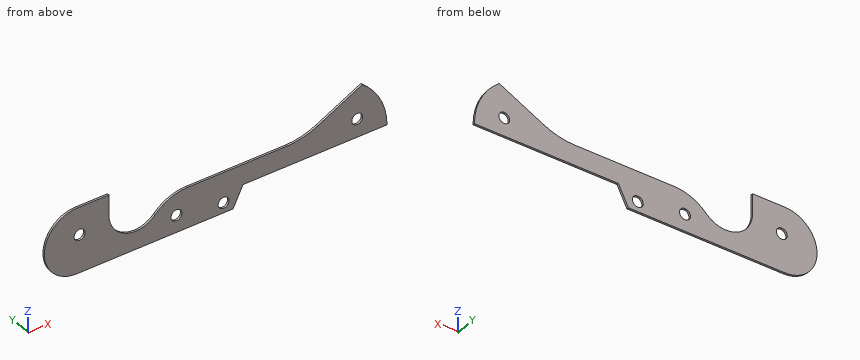
```python
from build123d import *

# Parameters (mm, degrees)
BOSS_EXTRUDE1_DEPTH = 0.508
SKETCH2_R           = 1.397
CUT_EXTRUDE1_DEPTH  = 1.508


with BuildPart() as part:
    # Sketch1 → Boss-Extrude1 (new body)
    with BuildSketch(Plane(origin=(0, 0, 0), x_dir=(1, 0, 0), z_dir=(0, 1, 0))):
        with BuildLine():
            Line((0, 8.255), (40.005, 8.255))
            Line((40.005, 8.255), (42.545, 3.175))
            Line((42.545, 3.175), (79.375, 3.175))
            ThreePointArc((79.375, 3.175), (77.699031657, -3.924515829), (73.025, -9.525))
            Line((73.025, -9.525), (61.684438597, -3.808211822))
            ThreePointArc((61.684438597, -3.808211822), (57.789960212, -2.38631827), (53.672063189, -1.905))
            Line((53.672063189, -1.905), (28.272063189, -1.905))
            ThreePointArc((28.272063189, -1.905), (23.804442177, -0.995706369), (20.047648696, 1.5875))
            ThreePointArc((20.047648696, 1.5875), (12.544893378, 3.184008757), (8.255, -3.175))
            Line((8.255, -3.175), (8.255, -8.255))
            Line((8.255, -8.255), (0, -8.255))
            ThreePointArc((0, -8.255), (-8.255, 0), (0, 8.255))
        make_face()
    extrude(amount=BOSS_EXTRUDE1_DEPTH)

    # Sketch2 → Cut-Extrude1 (cut, through all)
    with BuildSketch(Plane(origin=(0, 0.508, 0), x_dir=(1, 0, 0), z_dir=(0, 1, 0))):
        with Locations((0.762, -1.27)):
            Circle(SKETCH2_R)
        with Locations((25.527, 3.937)):
            Circle(SKETCH2_R)
        with Locations((37.592, 5.715)):
            Circle(SKETCH2_R)
        with Locations((71.755, -1.397)):
            Circle(SKETCH2_R)
    extrude(amount=-CUT_EXTRUDE1_DEPTH, mode=Mode.SUBTRACT)


solid = part.part
```
Source: CAD feature listing. Evaluate the final solid. Frame: model axes, mm. Coordinates: 2 decimals unless noted, no trailing zeros. Write each loop counter-clockwise with the first axis right and the second up, starting at its lowest first coordinate (ties: lowest second). Pieces come first, ordered by that corner, then holes. Notation, with made-up numbers: (81, 84) -> (127, 84) arc R13 cw to (127, 108) -> close; hole circle Ø7 at (45.25, -5). An arc over 180 degrees is marked (long way). Return JSON: item names as keys, results as strings. Group by question number.
1) Section query A-A, the plane z = 7. Return loops of the section in (x, y) (1 decimal), plus the area to 3 significant figures.
2) Section query C-C, the plane x = 29. Return loops of the section in (y, z) (3 decimals), plus the area to 3 significant figures.
3) Ray query, line 1 along X through (y, z) = (0.4, 1); line 2 along Z through (x, y) = (28, 0.05) (3 decimals); line 3 along X through (y, z) = (0.35, -3). Return the intervals inside material, ascending.
4) Contact query for a flat-ended pin moving along its axis: P1, Ø2, axis at x = 0.762, z = 1.27, coming from the +Y side (3 decimals). Output: stop coordinate, or through.
5) Section query D-D, the plane x = 41. Return loops of the section in (y, z) (3 decimals), plus the area to 3 significant figures.
6) Section query B-B, the plane y = 0.25. State how many separate pieces and enclosed holes the cut face has, plus the area to 3 significant figures.
From the geometry:
{
 "1": {"outline": "(-4.4, 0) -> (8.3, 0) -> (8.3, 0.5) -> (-4.4, 0.5) -> close; (68, 0) -> (75.7, 0) -> (75.7, 0.5) -> (68, 0.5) -> close", "area": "10.3 mm²"},
 "2": {"outline": "(0, -8.255) -> (0.508, -8.255) -> (0.508, 1.905) -> (0, 1.905) -> close", "area": "5.16 mm²"},
 "3": {"line 1": "-8.19 to -0.61, 2.13 to 8.61, 23.81 to 70.42, 73.09 to 78.82", "line 2": "-8.255 to 1.902", "line 3": "-7.69 to 12.13, 18.1 to 24.49, 26.56 to 79.37"},
 "4": {"P1": "through"},
 "5": {"outline": "(0, -6.265) -> (0.508, -6.265) -> (0.508, 1.905) -> (0, 1.905) -> close", "area": "4.15 mm²"},
 "6": {"separate pieces": "1", "enclosed holes": "4", "area": "769 mm²"}
}
